```python
from build123d import *

# Parameters (mm, degrees)
SKETCH1_W           = 95
SKETCH1_H           = 40
BOSS_EXTRUDE1_DEPTH = 20
BOSS_EXTRUDE3_DEPTH = 3
BOSS_EXTRUDE2_DEPTH = 20
SKETCH7_R           = 1.9
CUT_EXTRUDE5_DEPTH  = 100
BOSS_EXTRUDE4_DEPTH = 2
SKETCH10_R          = 10.5
CUT_EXTRUDE6_DEPTH  = 2
CUT_EXTRUDE7_REACH  = 20
SKETCH12_R          = 2
SKETCH12_R_2        = 1.5
SKETCH13_R          = 7.6
CUT_EXTRUDE9_DEPTH  = 1
CUT_EXTRUDE10_REACH = 41
SKETCH15_R          = 6.6
SKETCH16_R          = 2.6
CUT_EXTRUDE11_DEPTH = 14.9
SKETCH18_R          = 9.1
CUT_EXTRUDE12_DEPTH = 1
SKETCH19_R          = 8.1
CUT_EXTRUDE15_DEPTH = 34
SKETCH20_W          = 5.46
SKETCH20_H          = 1.201320344
CUT_EXTRUDE16_DEPTH = 22


with BuildPart() as part:
    # Sketch1 → Boss-Extrude1 (new body)
    with BuildSketch(Plane(origin=(0, 0, 0), x_dir=(1, 0, 0), z_dir=(0, 1, 0))):
        Rectangle(SKETCH1_W, SKETCH1_H)
    extrude(amount=BOSS_EXTRUDE1_DEPTH)

    # Sketch8 → Boss-Extrude2 (add)
    with BuildSketch(Plane(origin=(0, 0, 0), x_dir=(-1, 0, 0), z_dir=(0, -1, 0))):
        with BuildLine():
            Line((47.5, -20), (87.5, -20))
            ThreePointArc((87.5, -20), (107.5, 0), (87.5, 20))
            Line((87.5, 20), (47.5, 20))
            Line((47.5, 20), (47.5, -20))
        make_face()
        with BuildLine():
            Line((52.5, -15), (87.5, -15))
            ThreePointArc((87.5, -15), (102.5, 0), (87.5, 15))
            Line((87.5, 15), (52.5, 15))
            Line((52.5, 15), (52.5, -15))
        make_face(mode=Mode.SUBTRACT)
    extrude(amount=-BOSS_EXTRUDE2_DEPTH)

    # Sketch7 → Cut-Extrude5 (cut)
    with BuildSketch(Plane(origin=(47.5, 0, 0), x_dir=(0, 0, -1), z_dir=(1, 0, 0))):
        Polygon((-18.2, 13.064339828), (-20, 14.864339828), (-20, 5.134339828), (-18.2, 6.934339828), (-18.2, 4.499339828), (-16.56, 4.499339828), (-13.9, 7.159339828), (-13.9, 12.839339828), (-16.56, 15.499339828), (-18.2, 15.499339828), align=None)
        Polygon((-12.839339828, 13.9), (-7.159339828, 13.9), (-4.499339828, 16.56), (-4.499339828, 18.2), (-6.934339828, 18.2), (-5.134339828, 20), (-14.864339828, 20), (-13.064339828, 18.2), (-15.499339828, 18.2), (-15.499339828, 16.56), align=None)
        Polygon((-13.064339828, 1.798679656), (-14.863019485, 0), (-5.135660172, 0), (-6.934339828, 1.798679656), (-4.499339828, 1.798679656), (-4.499339828, 3.438679656), (-7.159339828, 6.098679656), (-12.839339828, 6.098679656), (-15.499339828, 3.438679656), (-15.499339828, 1.798679656), align=None)
        Polygon((14.864339828, 20), (5.134339828, 20), (6.934339828, 18.2), (4.499339828, 18.2), (4.499339828, 16.56), (7.159339828, 13.9), (12.839339828, 13.9), (15.499339828, 16.56), (15.499339828, 18.2), (13.064339828, 18.2), align=None)
        Polygon((5.135660172, 0), (14.863019485, 0), (13.064339828, 1.798679656), (15.499339828, 1.798679656), (15.499339828, 3.438679656), (12.839339828, 6.098679656), (7.159339828, 6.098679656), (4.499339828, 3.438679656), (4.499339828, 1.798679656), (6.934339828, 1.798679656), align=None)
        Polygon((20, 5.134339828), (20, 14.864339828), (18.2, 13.064339828), (18.2, 15.499339828), (16.56, 15.499339828), (13.9, 12.839339828), (13.9, 7.159339828), (16.56, 4.499339828), (18.2, 4.499339828), (18.2, 6.934339828), align=None)
        Polygon((6.098679656, 12.839339828), (6.098679656, 7.159339828), (2.73, 3.790660172), (2.73, 1.798679656), (-2.73, 1.798679656), (-2.73, 3.790660172), (-6.098679656, 7.159339828), (-6.098679656, 12.839339828), (-2.73, 16.208019485), (-2.73, 18.2), (2.73, 18.2), (2.73, 16.208019485), align=None)
        with Locations((-10, 10)):
            Circle(SKETCH7_R)
        with Locations((10, 10)):
            Circle(SKETCH7_R)
    extrude(amount=-CUT_EXTRUDE5_DEPTH, mode=Mode.SUBTRACT)



with BuildPart() as body_2:
    # Sketch8<3> → Boss-Extrude3 (new body)
    with BuildSketch(Plane(origin=(0, 0, 0), x_dir=(-1, 0, 0), z_dir=(0, -1, 0))):
        with BuildLine():
            Line((52.5, -15), (87.5, -15))
            ThreePointArc((87.5, -15), (102.5, 0), (87.5, 15))
            Line((87.5, 15), (52.5, 15))
            Line((52.5, 15), (52.5, -15))
        make_face()
    extrude(amount=-BOSS_EXTRUDE3_DEPTH)


with BuildPart() as part_1:
    add(part.part)

    add(body_2.part)  # Boss-Extrude4 merges body 2
    # Sketch9 → Boss-Extrude4 (add)
    with BuildSketch(Plane.ZY.offset(52.5)):
        Polygon((-15, 20), (-2.73, 20), (2.73, 20), (15, 20), (15, 3), (2.73, 3), (2.73, 3.790660172), (6.098679656, 7.159339828), (6.098679656, 12.839339828), (2.73, 16.208019485), (2.73, 18.2), (-2.73, 18.2), (-2.73, 16.208019485), (-6.098679656, 12.839339828), (-6.098679656, 7.159339828), (-2.73, 3.790660172), (-2.73, 3), (-15, 3), align=None)
    extrude(amount=BOSS_EXTRUDE4_DEPTH)

    # Sketch10 → Cut-Extrude6 (cut)
    with BuildSketch(Plane(origin=(0, 0, 0), x_dir=(-1, 0, 0), z_dir=(0, -1, 0))):
        with Locations((87.5, 0)):
            Circle(SKETCH10_R)
    extrude(amount=-CUT_EXTRUDE6_DEPTH, mode=Mode.SUBTRACT)

    # Sketch12 → Cut-Extrude7 (cut, up to next)
    with BuildSketch(Plane(origin=(0, 2, 0), x_dir=(-1, 0, 0), z_dir=(0, -1, 0)), mode=Mode.PRIVATE) as cut_extrude7_sk1:
        with Locations((87.5, 0)):
            Circle(SKETCH12_R)
    cut_extrude7_tool1 = extrude(cut_extrude7_sk1.sketch, amount=-CUT_EXTRUDE7_REACH, mode=Mode.PRIVATE) & part_1.part
    add(cut_extrude7_tool1.solids().sort_by_distance((-87.5, 2, 0))[0], mode=Mode.SUBTRACT)
    # Sketch12 → Cut-Extrude7 (cut, up to next)
    with BuildSketch(Plane(origin=(0, 2, 0), x_dir=(-1, 0, 0), z_dir=(0, -1, 0)), mode=Mode.PRIVATE) as cut_extrude7_sk2:
        with Locations((87.5, -7)):
            Circle(SKETCH12_R_2)
    cut_extrude7_tool2 = extrude(cut_extrude7_sk2.sketch, amount=-CUT_EXTRUDE7_REACH, mode=Mode.PRIVATE) & part_1.part
    add(cut_extrude7_tool2.solids().sort_by_distance((-87.5, 2, 7))[0], mode=Mode.SUBTRACT)
    # Sketch12 → Cut-Extrude7 (cut, up to next)
    with BuildSketch(Plane(origin=(0, 2, 0), x_dir=(-1, 0, 0), z_dir=(0, -1, 0)), mode=Mode.PRIVATE) as cut_extrude7_sk3:
        with Locations((80.5, 0)):
            Circle(SKETCH12_R_2)
    cut_extrude7_tool3 = extrude(cut_extrude7_sk3.sketch, amount=-CUT_EXTRUDE7_REACH, mode=Mode.PRIVATE) & part_1.part
    add(cut_extrude7_tool3.solids().sort_by_distance((-80.5, 2, 0))[0], mode=Mode.SUBTRACT)
    # Sketch12 → Cut-Extrude7 (cut, up to next)
    with BuildSketch(Plane(origin=(0, 2, 0), x_dir=(-1, 0, 0), z_dir=(0, -1, 0)), mode=Mode.PRIVATE) as cut_extrude7_sk4:
        with Locations((87.5, 7)):
            Circle(SKETCH12_R_2)
    cut_extrude7_tool4 = extrude(cut_extrude7_sk4.sketch, amount=-CUT_EXTRUDE7_REACH, mode=Mode.PRIVATE) & part_1.part
    add(cut_extrude7_tool4.solids().sort_by_distance((-87.5, 2, -7))[0], mode=Mode.SUBTRACT)
    # Sketch12 → Cut-Extrude7 (cut, up to next)
    with BuildSketch(Plane(origin=(0, 2, 0), x_dir=(-1, 0, 0), z_dir=(0, -1, 0)), mode=Mode.PRIVATE) as cut_extrude7_sk5:
        with Locations((94.5, 0)):
            Circle(SKETCH12_R_2)
    cut_extrude7_tool5 = extrude(cut_extrude7_sk5.sketch, amount=-CUT_EXTRUDE7_REACH, mode=Mode.PRIVATE) & part_1.part
    add(cut_extrude7_tool5.solids().sort_by_distance((-94.5, 2, 0))[0], mode=Mode.SUBTRACT)

    # Sketch13 → Cut-Extrude9 (cut)
    with BuildSketch(Plane.XY.offset(20)):
        with Locations((-66.5, 9.999339828)):
            Circle(SKETCH13_R)
    extrude(amount=-CUT_EXTRUDE9_DEPTH, mode=Mode.SUBTRACT)

    # Sketch15 → Cut-Extrude10 (cut, up to next)
    with BuildSketch(Plane.XY.offset(19), mode=Mode.PRIVATE) as cut_extrude10_sk1:
        with Locations((-66.5, 9.999339828)):
            Circle(SKETCH15_R)
    cut_extrude10_tool1 = extrude(cut_extrude10_sk1.sketch, amount=-CUT_EXTRUDE10_REACH, mode=Mode.PRIVATE) & part_1.part
    add(cut_extrude10_tool1.solids().sort_by_distance((-66.5, 9.99934, 19))[0], mode=Mode.SUBTRACT)

    # Sketch16 → Cut-Extrude11 (cut, through all)
    with BuildSketch(Plane(origin=(0, 13.9, 0), x_dir=(1, 0, 0), z_dir=(0, 1, 0))):
        with Locations((37.5, -9.999339828)):
            Circle(SKETCH16_R)
        with Locations((37.5, 9.999339828)):
            Circle(SKETCH16_R)
    extrude(amount=-CUT_EXTRUDE11_DEPTH, mode=Mode.SUBTRACT)

    # Sketch18 → Cut-Extrude12 (cut)
    with BuildSketch(Plane(origin=(0, 0, -20), x_dir=(-1, 0, 0), z_dir=(0, 0, -1))):
        with Locations((66.5, 9.999339828)):
            Circle(SKETCH18_R)
    extrude(amount=-CUT_EXTRUDE12_DEPTH, mode=Mode.SUBTRACT)

    # Sketch19 → Cut-Extrude15 (cut)
    with BuildSketch(Plane(origin=(0, 0, -19), x_dir=(-1, 0, 0), z_dir=(0, 0, -1))):
        with Locations((66.5, 9.999339828)):
            Circle(SKETCH19_R)
    extrude(amount=-CUT_EXTRUDE15_DEPTH, mode=Mode.SUBTRACT)

    # Sketch20 → Cut-Extrude16 (cut)
    with BuildSketch(Plane(origin=(-52.5, 0, 0), x_dir=(0, 0, -1), z_dir=(1, 0, 0))):
        with Locations((0, 2.399339828)):
            Rectangle(SKETCH20_W, SKETCH20_H)
    extrude(amount=-CUT_EXTRUDE16_DEPTH, mode=Mode.SUBTRACT)


solid = part_1.part
```
Work out the finished part from the listing and answer in its coordinate system (mm). A direction names the side the tool comes from. Round coordinates to 2 decimals unless told otherwise and drop trailing zeros. Write each loop counter-clockwise with the first axis right and the second up, starting at its lowest first coordinate (ties: lowest second). Pieces come first, ordered by that corner, then holes.
1) Which of the six approach directions +Z, -Z, +X, -X, +Y, -Y give full straight-line access (tool end or side, diameter ignored) to faces 1 (the face through (-2, 6.099, 10)), 2 (the face through (-7.769, 8.314, 9.123)), 3 (the face through (-2, 10, 13.9)), 4 (the face through (-2, 10, -13.9))?
2) Consider probe 1 along Z at (x, y) = (-87.5, 2.4); probe 2 along X at (y, z) = (2.75, 0); probe 3 along Z at (x, y) = (-9, 7.75). Determine where each line is inside the solid, lowest interval first.
3) A cutting plane is placed at D-D on x = 37.5. Give the number of separate pieces and of enclosed holes in the cut face, and give its area (3 significant figures).
4) A cutting plane is placed at B-B on x = -94.5. Determine the outline of the cut face in (y, z) (1 decimal), and give its area (3 significant figures).
5) Determine the mould class of faces 5 (the face through (-29, 0, 0)), 6 (the face through (-54.5, 17, 4)), 7 (the face through (-52.5, 10, 10)) for opening direction X: pulls with the +X half, pulls with the -X half, needs draft (parallel to the pull), parting line crosses it, or undercut.
6) Flat-ended cylindrical pins translate along their axes: P1, Ø1, axis at x = -55.5, z = 11, coming from the +Y side; P2, Ø0.7, axis at x = 4, z = 6, coming from the +Y side; P3, Ø0.7, axis at x = -12.5, z = -14, coming from the -Y side; P4, Ø1.8, axis at x = -87.5, z = -7, coming from the +Y side. Find the tip coordinate at first contact, or state that the pin passes through.
7) A cutting plane is placed at C-C on x = -69. Determine the outline of the cut face in (y, z), and give its area (3 significant figures).
8) A cutting plane is placed at A-A on z = 0. Determine the outline of the cut face in (x, y), and give its area (3 significant figures).
Entries:
1. face 1: +X, -Y
1. face 2: +X
1. face 3: +Z, +X
1. face 4: -Z, +X
2. probe 1: z = -20 to -8.5, -5.5 to -2, 2 to 5.5, 8.5 to 20
2. probe 2: x = -107.5 to -96, -93 to -89.5, -85.5 to -82, -79 to -74.5
2. probe 3: z = -13.9 to -6.1, 6.1 to 13.9
3. separate pieces: 3
3. enclosed holes: 1
3. area: 241 mm2
4. outline: (0, -18.7) - (20, -18.7) - (20, -13.3) - (3, -13.3) - (3, -1.5) - (2, -1.5) - (2, -7.8) - (0, -7.8) - close; (0, 7.8) - (2, 7.8) - (2, 1.5) - (3, 1.5) - (3, 13.3) - (20, 13.3) - (20, 18.7) - (0, 18.7) - close
4. area: 264 mm2
5. face 5: needs draft
5. face 6: undercut
5. face 7: pulls with the +X half
6. P1: stops at y = 3
6. P2: stops at y = 19.48
6. P3: stops at y = 0.51
6. P4: passes through
7. outline: (0, -20) - (1.25, -20) - (1.25, -19) - (2.29, -19) - (2.29, -2.73) - (1.8, -2.73) - (1.8, 2.73) - (2.29, 2.73) - (2.29, 15) - (3.89, 15) - (3.89, 19) - (2.82, 19) - (2.82, 20) - (0, 20) - close; (16.11, 15) - (20, 15) - (20, 20) - (17.18, 20) - (17.18, 19) - (16.11, 19) - close; (17.7, -19) - (18.75, -19) - (18.75, -20) - (20, -20) - (20, -15) - (17.7, -15) - close
7. area: 124 mm2
8. outline: (-107.5, 0) - (-98, 0) - (-98, 2) - (-96, 2) - (-96, 3) - (-102.5, 3) - (-102.5, 20) - (-107.5, 20) - close; (-93, 2) - (-89.5, 2) - (-89.5, 3) - (-93, 3) - close; (-85.5, 2) - (-82, 2) - (-82, 3) - (-85.5, 3) - close; (-79, 2) - (-77, 2) - (-77, 0) - (47.5, 0) - (47.5, 1.8) - (-74.5, 1.8) - (-74.5, 3) - (-79, 3) - close; (-54.5, 18.2) - (47.5, 18.2) - (47.5, 20) - (-54.5, 20) - close
8. area: 535 mm2
